For this review, use the dimensioned drawing (mm, ordinates from the lowest corner) and the shaded views. A direction names the side the tool comes from. Coordinates: 2 decimals unless noted, no trailing zeros. Order: outer loops, then holes, each group sorted by start corner. A loop starts at its lowest first (then second) coordinate and runs counter-clockwise, first axis right, second up. Notation, with made-up numbers: M 3.25,38 L 24.25,38 A26 cw 24.25,70 Z; hole C 89.25,59 d7. An arc over 180 degrees is marked long. Answer in a Markdown table with one row per item.
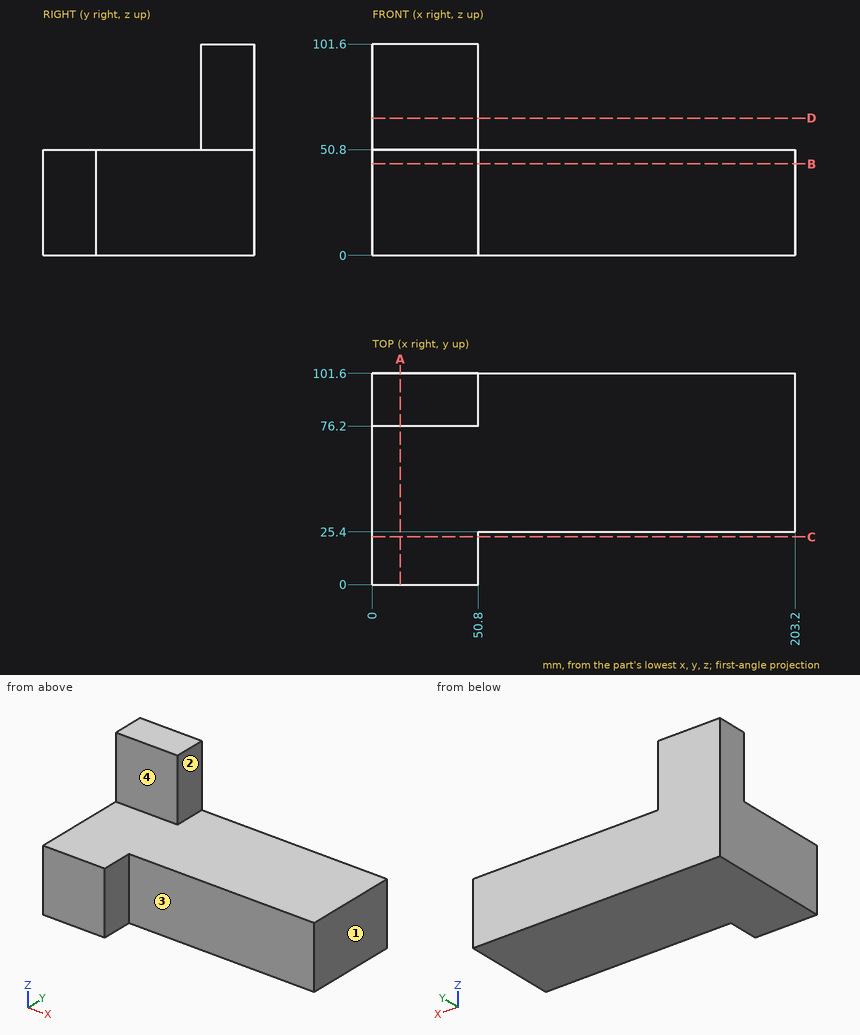
(1) For line 1 along Y through (x, z) = (20, 78); line 2 along Z through (x, y) = (43, 9); line 3 along Y through (x, z) = (98.5, 50), list the stretches that pass through material, from the lowest coordinate up. Write a range as from..to.
Return value:
| item | result |
|---|---|
| line 1 | y = 76.2..101.6 |
| line 2 | z = 0..50.8 |
| line 3 | y = 25.4..101.6 |
(2) Add section A-A, the plane x = 13.5. Give the boundary of the cut face in (y, z).
Return value:
| item | result |
|---|---|
| outline | M 0,0 L 101.6,0 L 101.6,101.6 L 76.2,101.6 L 76.2,50.8 L 0,50.8 Z |
(3) Insertion check: pin 1 Ø6 at (x, y) = (157, 74.5) entering from +Z. The pin has a flat end and moves straight along its axis. Give the tip position at first contact, or say it passes through.
Return value:
| item | result |
|---|---|
| pin 1 | stops at z = 50.8 |
(4) Add section B-B, the plane z = 44. Give the boundary of the cut face in (x, y), and give its area (3 significant figures).
Return value:
| item | result |
|---|---|
| outline | M 0,0 L 50.8,0 L 50.8,25.4 L 203.2,25.4 L 203.2,101.6 L 0,101.6 Z |
| area | 16,800 mm2 |
(5) For the marked faces 1, 2, 3 and 4, list the 3-axis set-ups (+Z, -Z, +X, -X, +Y, -Y) from which the entire face can be reached by the end or side of a thin tool; tool diameter is ignored.
Return value:
| item | result |
|---|---|
| face 1 | +Z, -Z, +X, +Y, -Y |
| face 2 | +Z, +X, +Y, -Y |
| face 3 | +Z, -Z, +X, -Y |
| face 4 | +Z, +X, -X, -Y |
(6) Add section C-C, the plane y = 23. Give the boundary of the cut face in (x, z).
Return value:
| item | result |
|---|---|
| outline | M 0,0 L 50.8,0 L 50.8,50.8 L 0,50.8 Z |
(7) Add section D-D, the plane z = 66. Give the boundary of the cut face in (x, y).
Return value:
| item | result |
|---|---|
| outline | M 0,76.2 L 50.8,76.2 L 50.8,101.6 L 0,101.6 Z |
